```python
from build123d import *

# Parameters (mm, degrees)
BOSS_EXTRUDE1_DEPTH       = 4
F_2_0MM_DOWEL_HOLE1_D     = 18
F_2_0MM_DOWEL_HOLE2_D     = 2
F_2_0MM_DOWEL_HOLE2_DEPTH = 10
CUT_EXTRUDE3_DEPTH        = 2


with BuildPart() as part:
    # Sketch1 → Boss-Extrude1 (new body)
    with BuildSketch(Plane(origin=(0, 0, 0), x_dir=(1, 0, 0), z_dir=(0, 1, 0))):
        with BuildLine():
            Line((16.549446177, 5.7), (18.037708346, 5.7))
            ThreePointArc((18.037708346, 5.7), (21.573242252, 4.235533906), (23.037708346, 0.7))
            Line((23.037708346, 0.7), (23.037708346, -11.514786255))
            ThreePointArc((23.037708346, -11.514786255), (22.744815127, -12.221893036), (22.037708346, -12.514786255))
            Line((22.037708346, -12.514786255), (-22, -12.514786255))
            ThreePointArc((-22, -12.514786255), (-22.707106781, -12.221893036), (-23, -11.514786255))
            Line((-23, -11.514786255), (-23, 0.7))
            ThreePointArc((-23, 0.7), (-21.535533906, 4.235533906), (-18, 5.7))
            Line((-18, 5.7), (-16.549446177, 5.7))
            ThreePointArc((-16.549446177, 5.7), (0, 12.280701177), (16.549446177, 5.7))
        make_face()
    extrude(amount=BOSS_EXTRUDE1_DEPTH)

    # Ø2.0mm Dowel Hole1 (through all)
    with Locations(Plane(origin=(0, 4, 0), x_dir=(1, 0, 0), z_dir=(0, 1, 0))):
        with Locations((0, -1.235213745)):
            Hole(F_2_0MM_DOWEL_HOLE1_D / 2)

    # Ø2.0mm Dowel Hole2
    with Locations(Plane(origin=(0, 4, 0), x_dir=(1, 0, 0), z_dir=(0, 1, 0))):
        with Locations((-19.65, -1.014786255), (19.65, -1.014786255)):
            Hole(F_2_0MM_DOWEL_HOLE2_D / 2, depth=F_2_0MM_DOWEL_HOLE2_DEPTH)

    # Sketch9 → Cut-Extrude3 (cut)
    with BuildSketch(Plane(origin=(0, 4, 0), x_dir=(1, 0, 0), z_dir=(0, 1, 0))):
        with BuildLine():
            Line((-8.5, 9.264786255), (8.5, 9.264786255))
            ThreePointArc((8.5, 9.264786255), (13.449747468, 7.214533723), (15.5, 2.264786255))
            Line((15.5, 2.264786255), (15.5, -5.735213745))
            ThreePointArc((15.5, -5.735213745), (13.742640687, -9.977854433), (9.5, -11.735213745))
            Line((9.5, -11.735213745), (-9.5, -11.735213745))
            ThreePointArc((-9.5, -11.735213745), (-13.742640687, -9.977854433), (-15.5, -5.735213745))
            Line((-15.5, -5.735213745), (-15.5, 2.264786255))
            ThreePointArc((-15.5, 2.264786255), (-13.449747468, 7.214533723), (-8.5, 9.264786255))
        make_face()
    extrude(amount=-CUT_EXTRUDE3_DEPTH, mode=Mode.SUBTRACT)


solid = part.part
```
Geometry check sheet. Reference: the model listing, model coordinates, mm. A direction names the side the tool comes from. Give positions to 0.01 mm unless a question says otherwise; leave off trailing zeros. Write each loop counter-clockwise with the first axis right and the second up, starting at its lowest first coordinate (ties: lowest second). Pieces come first, ordered by that corner, then holes. Notation, with made-up numbers: (87.5, 52) - (129.5, 52) arc R17 cw to (129.5, 77) - close; hole circle Ø10 at (10.25, 26.5). An arc over 180 degrees is marked (long way). Use a Markdown table: item, result.
Q1. Draft check along X on faces 1 (the face through (-21.57, 1.97, -4.2)), 2 (the face through (0, 2, 12.515)), 3 (the face through (-13.7, 3.01, 10.02)). Enter one of: pulls with the +X half, pulls with the -X half, needs draft (parallel to the pull), parting line crosses it, or undercut.
Computed:
| item | result |
|---|---|
| face 1 | pulls with the -X half |
| face 2 | needs draft |
| face 3 | undercut |
Q2. Section check B-B, the plane z = 9. Enter the section's corners in (x, y).
Computed:
| item | result |
|---|---|
| outline | (-23, 0) - (-4.55, 0) - (-4.55, 2) - (-14.53, 2) - (-14.53, 4) - (-23, 4) - close; (4.55, 0) - (23.04, 0) - (23.04, 4) - (14.53, 4) - (14.53, 2) - (4.55, 2) - close |
Q3. Section check C-C, the plane x = -12.5. Enter the section's corners in (y, z).
Computed:
| item | result |
|---|---|
| outline | (0, -8.79) - (4, -8.79) - (4, -8.01) - (2, -8.01) - (2, 10.93) - (4, 10.93) - (4, 12.51) - (0, 12.51) - close |
Q4. Section check D-D, the plane y = 0.7. Enter the section's corners in (x, z), then the cut area to 3 significant figures.
Computed:
| item | result |
|---|---|
| outline | (-23, -0.7) arc R5 ccw to (-18, -5.7) - (-16.55, -5.7) arc R24.1 ccw to (16.55, -5.7) - (18.04, -5.7) arc R5 ccw to (23.04, -0.7) - (23.04, 11.51) arc R1 ccw to (22.04, 12.51) - (-22, 12.51) arc R1 ccw to (-23, 11.51) - close; hole circle Ø2 at (-19.65, 1.01); hole circle Ø18 at (0, 1.24); hole circle Ø2 at (19.65, 1.01) |
| area | 716 mm² |
Q5. Section check A-A, the plane x = 0. Enter the section's corners in (y, z).
Computed:
| item | result |
|---|---|
| outline | (0, -12.28) - (4, -12.28) - (4, -9.26) - (2, -9.26) - (2, -7.76) - (0, -7.76) - close; (0, 10.24) - (2, 10.24) - (2, 11.74) - (4, 11.74) - (4, 12.51) - (0, 12.51) - close |
Q6. Set-up check for faces 4 (the face through (0, 3, -9.265)), 5 (the face through (-17, 2, -5.7)), 6 (the face through (0, 4, 12)): record each of +Z, -Z, +X, -X, +Y, -Y from which the full face is reachable in a straight line by a thin tool's end or side.
Computed:
| item | result |
|---|---|
| face 4 | +Y |
| face 5 | -Z, -X, +Y, -Y |
| face 6 | +Z, -Z, +X, -X, +Y |
Q7. Go/stop test with flat-tipped pins: P1, Ø0.7, axis at x = 17, y = 1, coming from the -Z side; P2, Ø3, axis at x = 12.5, z = -1, coming from the +Y side; P3, Ø0.6, axis at x = -3.5, y = 3, coming from the -Z side. Record where each tip stops, or that it passes through.
Computed:
| item | result |
|---|---|
| P1 | stops at z = -5.7 |
| P2 | stops at y = 2 |
| P3 | stops at z = -12.07 |
Q8. Thickness scan on L1, parallel to Z at x = 0, y = 1.2; L2, parallel to Y at x = 11, z = -2; L3, parallel to X at y = 0.6, z = -6.5. Record the ranges inside material, lowest first. Write a range as [from, to].
Computed:
| item | result |
|---|---|
| L1 | z = [-12.28, -7.76], [10.24, 12.51] |
| L2 | y = [0, 2] |
| L3 | x = [-15.66, -4.6], [4.6, 15.66] |
